CAD build for the part. Positions are in the model's coordinates, mm. Face numbers are marked on the shaded views. A direction names the side the tool comes from. Give positions to 0.01 mm unless a question says otherwise; leave off trailing zeros. Write each loop counter-clockwise with the first axis right and the second up, starting at its lowest first coordinate (ties: lowest second). Pieces come first, ordered by that corner, then holes. Notation, with made-up numbers: M 86,-16.75 L 122,-16.75 A17 ccw 122,15.25 Z; hole C 52,8 d8. An arc over 180 degrees is marked long. One line per question, with ' | ' between items. Start each with the question number.
1. Cut at A-A, the plane x = 15.5. Write the cut outline in (y, z).
2. Which spindle directions (+Z, -Z, +X, -X, +Y, -Y) get a long thin tool onto all of the face, cutting with end or side? Do the marked faces 1, 2 and 3. Say none if no direction does.
3. Cut at B-B, the plane z = 0. Write the cut outline in (x, y), then the cut area to 3 significant figures.
4. Cut at D-D, the plane z = 31.5. Write the cut outline in (x, y).
5. Flat gauge pins, fed straight in: pin 1 (3 mm diameter, centred on x = 9, z = 16, fed in from -Y); pin 2 (1.5 mm diameter, centred on y = 3.5, z = -7, fed in from -X); pin 3 (1 mm diameter, centred on y = 0.5, z = 21.5, fed in from -X); pin 4 (1.5 mm diameter, centred on x = 12, y = 3, fed in from +Z). Where does each tip first touch, or does it go through?
6. Wall check: L1, parallel to Z at x = -15.5, y = 3.65; L2, parallel to X at y = 1.95, z = 0; L3, parallel to X at y = 3.2, z = 15.5. Give the ranges that are in metal, low to high.
7. Cut at C-C, the plane x = -31.5. Write the cut outline in (y, z), then the cut area to 3 significant figures.
```python
from build123d import *

# Parameters (mm, degrees)
CROQUIS1_R              = 1.7
SALIENTE_EXTRUIR1_DEPTH = 5


with BuildPart() as part:
    # Croquis1 → Saliente-Extruir1 (new body)
    with BuildSketch(Plane(origin=(0, 0, 0), x_dir=(1, 0, 0), z_dir=(0, 1, 0))):
        Polygon((-35, 4), (-20, 4), (-20, 19), (20, 19), (20, 4), (35, 4), (35, -4), (20, -4), (20, -19), (4, -19), (4, -34), (-4, -34), (-4, -19), (-20, -19), (-20, -4), (-35, -4), align=None)
        with Locations((-15.5, 15.5)):
            Circle(CROQUIS1_R, mode=Mode.SUBTRACT)
        with Locations((15.5, 15.5)):
            Circle(CROQUIS1_R, mode=Mode.SUBTRACT)
        with Locations((15.5, -15.5)):
            Circle(CROQUIS1_R, mode=Mode.SUBTRACT)
        with Locations((-15.5, -15.5)):
            Circle(CROQUIS1_R, mode=Mode.SUBTRACT)
        with Locations((-31.5, 0)):
            Circle(CROQUIS1_R, mode=Mode.SUBTRACT)
        with Locations((0, -31.5)):
            Circle(CROQUIS1_R, mode=Mode.SUBTRACT)
        with Locations((31.5, 0)):
            Circle(CROQUIS1_R, mode=Mode.SUBTRACT)
    extrude(amount=SALIENTE_EXTRUIR1_DEPTH)


solid = part.part
```
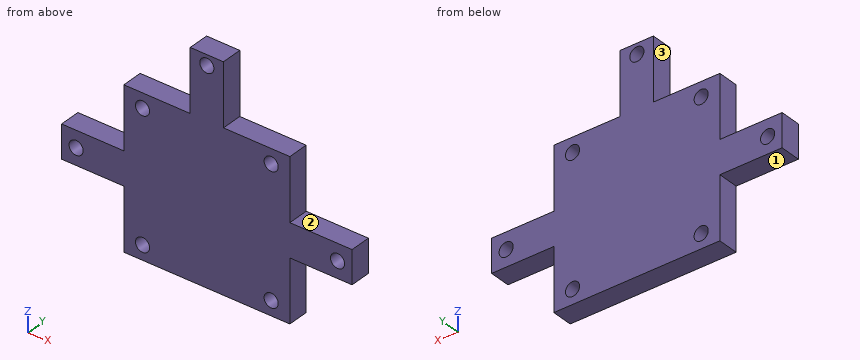
Here are the results:
1) outline: M 0,-19 L 5,-19 L 5,-17.2 L 0,-17.2 Z; M 0,-13.8 L 5,-13.8 L 5,13.8 L 0,13.8 Z; M 0,17.2 L 5,17.2 L 5,19 L 0,19 Z
2) face 1: -Z, -X, +Y, -Y | face 2: +Z, +X, +Y, -Y | face 3: +Z, -X, +Y, -Y
3) outline: M -35,0 L -33.2,0 L -33.2,5 L -35,5 Z; M -29.8,0 L 29.8,0 L 29.8,5 L -29.8,5 Z; M 33.2,0 L 35,0 L 35,5 L 33.2,5 Z | area: 316 mm^2
4) outline: M -4,0 L -1.7,0 L -1.7,5 L -4,5 Z; M 1.7,0 L 4,0 L 4,5 L 1.7,5 Z
5) pin 1: y = 0 | pin 2: x = -20 | pin 3: x = -4 | pin 4: z = 19
6) L1: -19 to -17.2, -13.8 to 13.8, 17.2 to 19 | L2: -35 to -33.2, -29.8 to 29.8, 33.2 to 35 | L3: -20 to -17.2, -13.8 to 13.8, 17.2 to 20
7) outline: M 0,-4 L 5,-4 L 5,-1.7 L 0,-1.7 Z; M 0,1.7 L 5,1.7 L 5,4 L 0,4 Z | area: 23.0 mm^2
